Read the model definition and answer for the solid it produces. Units are mm, in the model's axes. A direction names the side the tool comes from. Coordinates: 2 decimals unless noted, no trailing zeros. Order: outer loops, then holes, each group sorted by start corner. A loop starts at its lowest first (then second) coordinate and runs counter-clockwise, first axis right, second up. Notation, with made-up numbers: (16, 13) - (45, 13) arc R30 ccw to (45, 50) - close; hole circle Ø11 at (36, 55). An arc over 180 degrees is marked (long way). Answer as a JSON object with one key per item and string values. Group by question number.
from build123d import *

# Parameters (mm, degrees)
F0_W     = 43
F0_H     = 43
F1_DEPTH = 40
F2_R     = 2.5
F3_DEPTH = 24
F4_SIZE  = 5


with BuildPart() as f1:
    # F0 (on Top) → F1 (new body)
    with BuildSketch(Plane.XY):
        Rectangle(F0_W, F0_H)
    extrude(amount=F1_DEPTH)

    # F2 (on face) → F3 (join)
    with BuildSketch(Plane.XY.offset(40)):
        Circle(F2_R)
    extrude(amount=F3_DEPTH)

    # F4
    f4_edges = [f1.edges().sort_by_distance(p)[0] for p in [
        (-21.5, -21.5, 20),
        (21.5, -21.5, 20),
        (21.5, 21.5, 20),
        (-21.5, 21.5, 20),
    ]]
    chamfer(f4_edges, length=F4_SIZE)


solid = f1.part
1. Straight lines are drawn through the part: L1, parallel to Z at x = 17.5, y = 15; L2, parallel to Y at x = 19, z = 30.5; L3, parallel to X at y = 18, z = 22.5. For each, find the intervals that lie inside material, in ascending order.
2. Given pin 1 (3 mm diameter, centred on y = 5, z = 54, fed in from -X); pin 2 (5 mm diameter, centred on x = -9.5, y = -13.5, fed in from +Z); pin 3 (3 mm diameter, centred on x = -13.5, y = 3.5, fed in from -Z), each flat-ended and moving along its own axis, determine where each tip first touches the part or whether it passes through.
3. A cutting plane is placed at A-A on y = 0. Write down the section's boundary in (x, z).
4. For faces 1 (the cylindrical face through (-0.54, -2.44, 51.83)), 2 (the flat face through (-19, -19, 20)), determine the directions among +Z, -Z, +X, -X, +Y, -Y from which every point of the face is accessible in a straight line to the end or side of a thin tool.
5. A cutting plane is placed at D-D on y = 18.5. Write down the section's boundary in (x, z), and give its area (3 significant figures).
6. A cutting plane is placed at C-C on x = 9. Write down the section's boundary in (y, z), and give its area (3 significant figures).
Derived:
{
 "1": {"L1": "z = 0 to 40", "L2": "y = -19 to 19", "L3": "x = -20 to 20"},
 "2": {"pin 1": "passes through", "pin 2": "stops at z = 40", "pin 3": "stops at z = 0"},
 "3": {"outline": "(-21.5, 0) - (21.5, 0) - (21.5, 40) - (2.5, 40) - (2.5, 64) - (-2.5, 64) - (-2.5, 40) - (-21.5, 40) - close"},
 "4": {"face 1": "+Z", "face 2": "+Z, -Z, -X, -Y"},
 "5": {"outline": "(-19.5, 0) - (19.5, 0) - (19.5, 40) - (-19.5, 40) - close", "area": "1,560 mm2"},
 "6": {"outline": "(-21.5, 0) - (21.5, 0) - (21.5, 40) - (-21.5, 40) - close", "area": "1,720 mm2"}
}
